Here's how the part is built. I have some questions about the finished solid (model axes, mm). Round coordinates to 2 decimals unless told otherwise and drop trailing zeros. Loops run counter-clockwise (first coordinate to the right, second up) from the corner with the lowest first, then second, coordinate; pieces in that order, holes last. Notation, with made-up numbers: M 37.25,-31 L 65.25,-31 A23 cw 65.25,-12 Z; hole C 55,-4.5 d6. An arc over 180 degrees is marked long. Answer as a JSON object with one key per item and string values.
from build123d import *

# Parameters (mm, degrees)
SKETCH1_R                                        = 45.466
BOSS_EXTRUDE1_DEPTH                              = 25.4
SKETCH3_R                                        = 20.32
CUT_EXTRUDE1_DEPTH                               = 12.7
CSK_FOR_1_4_FLAT_HEAD_MACHINE_SCREW1_D           = 6.5278
CSK_FOR_1_4_FLAT_HEAD_MACHINE_SCREW1_DEPTH       = 25.4
CSK_FOR_1_4_FLAT_HEAD_MACHINE_SCREW1_CSINK_D     = 12.8778
CSK_FOR_1_4_FLAT_HEAD_MACHINE_SCREW1_CSINK_ANGLE = 82
CSK_FOR_1_4_FLAT_HEAD_MACHINE_SCREW1_TIP         = 1.961148974
SKETCH9_R                                        = 53.031918303
CUT_EXTRUDE3_DEPTH                               = 12.7


with BuildPart() as part:
    # Sketch1 → Boss-Extrude1 (new body)
    with BuildSketch(Plane(origin=(0, 0, 0), x_dir=(1, 0, 0), z_dir=(0, 1, 0))):
        Circle(SKETCH1_R)
    extrude(amount=BOSS_EXTRUDE1_DEPTH)

    # Sketch3 → Cut-Extrude1 (cut)
    with BuildSketch(Plane.XZ):
        Circle(SKETCH3_R)
    extrude(amount=-CUT_EXTRUDE1_DEPTH, mode=Mode.SUBTRACT)

    # CSK for 1/4 Flat Head Machine Screw1
    with Locations(Plane(origin=(0, 25.4, 0), x_dir=(1, 0, 0), z_dir=(0, 1, 0))):
        with Locations((0, 0)):
            CounterSinkHole(CSK_FOR_1_4_FLAT_HEAD_MACHINE_SCREW1_D / 2, CSK_FOR_1_4_FLAT_HEAD_MACHINE_SCREW1_CSINK_D / 2, depth=CSK_FOR_1_4_FLAT_HEAD_MACHINE_SCREW1_DEPTH, counter_sink_angle=CSK_FOR_1_4_FLAT_HEAD_MACHINE_SCREW1_CSINK_ANGLE)
            with Locations((0, 0, -(CSK_FOR_1_4_FLAT_HEAD_MACHINE_SCREW1_DEPTH + CSK_FOR_1_4_FLAT_HEAD_MACHINE_SCREW1_TIP / 2))):  # 118° drill point
                Cone(0, CSK_FOR_1_4_FLAT_HEAD_MACHINE_SCREW1_D / 2, CSK_FOR_1_4_FLAT_HEAD_MACHINE_SCREW1_TIP, mode=Mode.SUBTRACT)

    # Sketch9 → Cut-Extrude3 (cut)
    with BuildSketch(Plane.XZ):
        Circle(SKETCH9_R)
    extrude(amount=-CUT_EXTRUDE3_DEPTH, mode=Mode.SUBTRACT)


solid = part.part
Item 1: I want a section at D-D on z = 28. List the corners of the cut face in (x, y) for me, plus the area to 3 significant figures.
Solution:
{"outline": "M -35.82,12.7 L 35.82,12.7 L 35.82,25.4 L -35.82,25.4 Z", "area": "910 mm2"}
Item 2: If I drill on L1, parallel to Z at x = 0, y = 15; L2, parallel to X at y = 19, z = -33.5; L3, parallel to X at y = 17.25, z = -8, over which ranges is the centre line in solid material (lowest first)? Write a range as from..to.
Solution:
{"L1": "z = -45.47..-3.26, 3.26..45.47", "L2": "x = -30.74..30.74", "L3": "x = -44.76..44.76"}
Item 3: We'd pull the mould along Z, two halves only. Please class faces 1 (the face through (-9.856, 18.961, 44.385)), 2 (the face through (0.741, 21.925, 3.337)), 3 (the face through (9, 25.4, -1)): +Z half, -Z half, draft (parallel to the pull), parting line (faces both ways), or undercut.
Solution:
{"face 1": "parting line", "face 2": "undercut", "face 3": "draft"}
Item 4: I want a section at C-C on y = 17.5. List the corners of the cut face in (x, z) for me, plus the area to 3 significant figures.
Solution:
{"outline": "C 0,0 d90.93; hole C 0,0 d6.53", "area": "6,460 mm2"}
Item 5: I want a section at B-B on x = 0. List the corners of the cut face in (y, z) for me, plus the area to 3 significant figures.
Solution:
{"outline": "M 12.7,-45.47 L 25.4,-45.47 L 25.4,-6.44 L 21.75,-3.26 L 12.7,-3.26 Z; M 12.7,3.26 L 21.75,3.26 L 25.4,6.44 L 25.4,45.47 L 12.7,45.47 Z", "area": "1,060 mm2"}
Item 6: I want a section at A-A on z = 0. List the corners of the cut face in (x, y) for me.
Solution:
{"outline": "M -45.47,12.7 L -3.26,12.7 L -3.26,21.75 L -6.44,25.4 L -45.47,25.4 Z; M 3.26,12.7 L 45.47,12.7 L 45.47,25.4 L 6.44,25.4 L 3.26,21.75 Z"}
Item 7: For P1, Ø3, axis at y = 23.5, z = 7, coming from the +X side; P2, Ø5, axis at y = 19, z = -14, coming from the +X side; P3, Ø3, axis at y = 20, z = 15, coming from the +X side, each with a flat end and sliding along its axis, tell me the tip position at first contact or that it passes through.
Solution:
{"P1": "stops at x = 45.13", "P2": "stops at x = 43.99", "P3": "stops at x = 43.42"}
